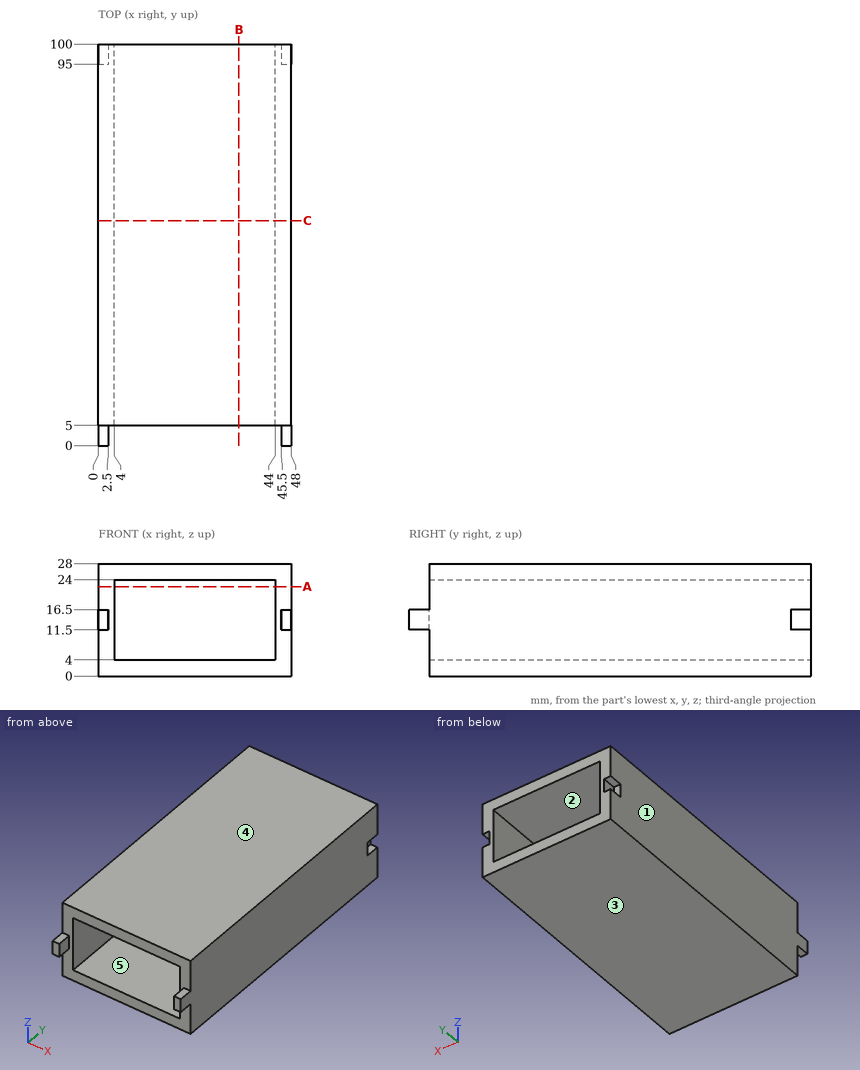
Geometry check sheet. Reference: drawing and pictorial views, mm from the part's lowest x, y, z. A direction names the side the tool comes from. Coordinates: 2 decimals unless noted, no trailing zeros. Order: outer loops, then holes, each group sorted by start corner. A loop starts at its lowest first (then second) coordinate and runs counter-clockwise, first axis right, second up.
Item 1: Section check A-A, the plane z = 22.25. Enter the section's corners in (x, y), then the cut area to 3 significant figures.
Filled in:
outline: (0, 5) - (4, 5) - (4, 100) - (0, 100) - close; (44, 5) - (48, 5) - (48, 100) - (44, 100) - close
area: 760 mm2
Item 2: Section check B-B, the plane x = 35. Enter the section's corners in (y, z), then the cut area to 3 significant figures.
Filled in:
outline: (5, 0) - (100, 0) - (100, 4) - (5, 4) - close; (5, 24) - (100, 24) - (100, 28) - (5, 28) - close
area: 760 mm2
Item 3: Depth check by flat-ended pin: pin 1 (2.5 mm diameter, centred on y = 97.5, z = 14.5, fed in from +X); pin 2 (2 mm diameter, centred on y = 62, z = 8, fed in from -X); pin 3 (3 mm diameter, centred on x = 1, y = 3, fed in from +Z); pin 4 (0.8 mm diameter, centred on x = 1, y = 3, fed in from -Z). Enter the tip coordinate at first touch or a pass-through.
Filled in:
pin 1: stops at x = 45.5
pin 2: stops at x = 0
pin 3: stops at z = 16.5
pin 4: stops at z = 11.5
Item 4: Material ranges on L1, parallel to X at y = 68, z = 7; L2, parallel to Z at x = 35.5, y = 30.5; L3, parallel to X at y = 95.5, z = 15.75, recorded low to high.
Filled in:
L1: x = 0 to 4, 44 to 48
L2: z = 0 to 4, 24 to 28
L3: x = 2.5 to 4, 44 to 45.5
Item 5: Access from +Z, -Z, +X, -X, +Y, -Y to the whole of each face (thin tool, end or side, straight path). Record for the marked faces 4 and 5.
Filled in:
face 4: +Z, +X, -X, +Y, -Y
face 5: +Y, -Y
Item 6: Section check C-C, the plane y = 56. Enter the section's corners in (x, z), then the cut area to 3 significant figures.
Filled in:
outline: (0, 0) - (48, 0) - (48, 28) - (0, 28) - close; hole (4, 4) - (44, 4) - (44, 24) - (4, 24) - close
area: 544 mm2
Item 7: Release check for a two-part mould opening along X. For the marked faces 1, 2 and 3 record: +X half, -X half, draft (parallel to the pull), parting line (faces both ways), or undercut.
Filled in:
face 1: -X half
face 2: undercut
face 3: draft
